Can you work these out from the drawing? Everything is in mm from the part's minimum corner. A direction names the side the tool comes from. Round coordinates to 2 decimals unless told otherwise and drop trailing zeros. Loops run counter-clockwise (first coordinate to the right, second up) from the corner with the lowest first, then second, coordinate; pieces in that order, holes last. Notation, with made-up numbers: (4, 25.25) -> (34, 25.25) arc R23 ccw to (34, 40.25) -> close; hole circle Ø11 at (39.25, 1.25). An arc over 180 degrees is marked (long way). One line per item, written item: value.
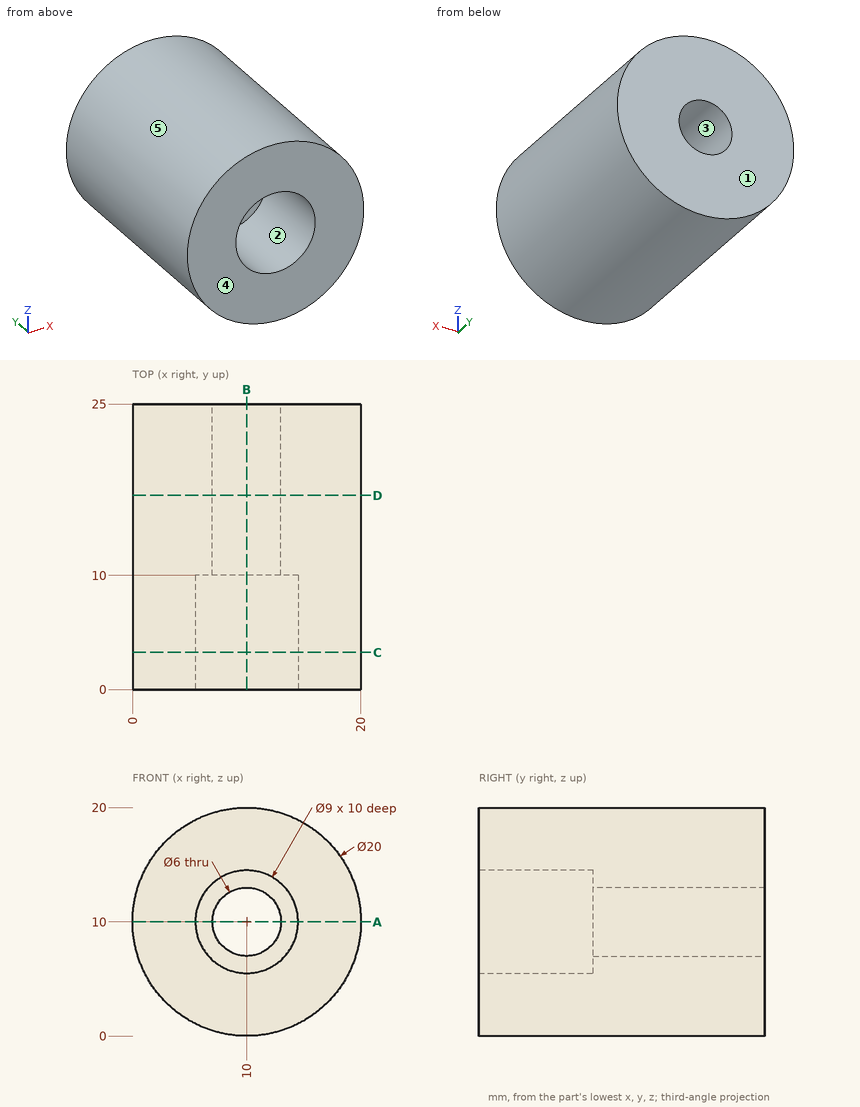
(1) Imagine slicing it at D-D on y = 17. Write out the boundary of the cut face in (x, z), then the cut area to 3 significant figures.
Results below:
outline: circle Ø20 at (10, 10); hole circle Ø6 at (10, 10)
area: 286 mm²
(2) Imagine slicing it at B-B on x = 10. Write out the boundary of the cut face in (y, z).
Results below:
outline: (0, 0) -> (25, 0) -> (25, 7) -> (10, 7) -> (10, 5.5) -> (0, 5.5) -> close; (0, 14.5) -> (10, 14.5) -> (10, 13) -> (25, 13) -> (25, 20) -> (0, 20) -> close
(3) Please list where these lines run through material, in increasing order: L1, parallel to X at y = 5.5, z = 10; L2, parallel to X at y = 19.25, z = 10; L3, parallel to Y at x = 10.5, z = 5.75.
Results below:
L1: x = 0 to 5.5, 14.5 to 20
L2: x = 0 to 7, 13 to 20
L3: y = 10 to 25
(4) On a 3-axis mill with a long thin cutter (end or side, diameter ignored), from which of +Z, -Z, +X, -X, +Y, -Y can I reach the whole of each face in a straight line? I mean the marked faces 1 and 2. Say none if no direction works.
Results below:
face 1: +Z, -Z, +X, -X, +Y
face 2: -Y
(5) We'd pull the mould along Z, two halves only. Please class the marked faces 3, 4 and 5: +Z half, -Z half, draft (parallel to the pull), parting line (faces both ways), or undercut.
Results below:
face 3: undercut
face 4: draft
face 5: parting line
(6) For pin 1 Ø5 at (y, z) = (18.5, 2.5) entering from -X; pin 2 Ø8 at (x, z) = (10, 10) entering from -Y; pin 3 Ø2 at (y, z) = (15, 12) entering from -X, each with a flat end and sliding along its axis, tell me the tip position at first contact or that it passes through.
Results below:
pin 1: stops at x = 1.34
pin 2: stops at y = 10
pin 3: stops at x = 0.05
(7) Imagine slicing it at A-A on z = 10. Write out the boundary of the cut face in (x, y), then the cut area to 3 significant figures.
Results below:
outline: (0, 0) -> (5.5, 0) -> (5.5, 10) -> (7, 10) -> (7, 25) -> (0, 25) -> close; (13, 10) -> (14.5, 10) -> (14.5, 0) -> (20, 0) -> (20, 25) -> (13, 25) -> close
area: 320 mm²
(8) Imagine slicing it at C-C on y = 3.25. Write out the boundary of the cut face in (x, z), then the cut area to 3 significant figures.
Results below:
outline: circle Ø20 at (10, 10); hole circle Ø9 at (10, 10)
area: 251 mm²
